Source: three-view drawing plus pictorial views. Frame: mm from the lowest corner of the part. A direction names the side the tool comes from. Coordinates: 2 decimals unless noted, no trailing zeros. Loops run counter-clockwise (first coordinate to the right, second up) from the corner with the lowest first, then second, coordinate; pieces in that order, holes last. Notation, with made-up numbers: (60, 74) - (91, 74) arc R13 ccw to (91, 94) - close; hole circle Ø4 at (42.25, 39). An arc over 180 degrees is marked (long way). Use CSV: the item, a comma, the result in double quotes. Start each with the question number.
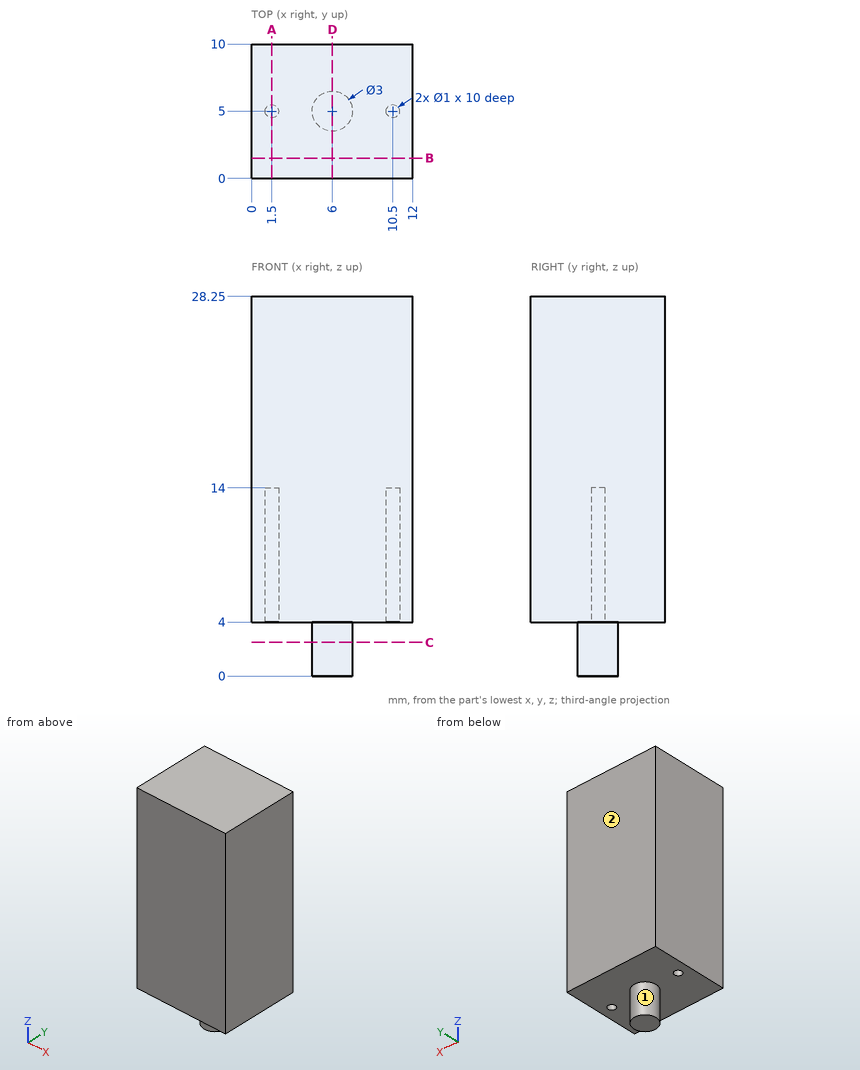
(1) Section A-A on x = 1.5. Output: boundary loops of the cut face in (y, z).
(2) Ray query, line 1 (Y direction, x = 1.5, z = 7.25); line 2 (Z direction, x = 8.5, y = 3.25); line 3 (Z direction, x = 10.25, y = 5). Return the intervals inside material, ascending. Write a range as [from, to].
(3) Pin query (flat end, axial travel): pin 1 Ø1 at (x, y) = (4.5, 3) entering from -Z; pin 2 Ø0.8 at (x, y) = (1.5, 5) entering from -Z. Return the tip coordinate at first contact, or that it passes through.
(4) Reachability of the marked faces 1 and 2 from +Z, -Z, +X, -X, +Y, -Y: full face, straight path, thin tool, end or side. Return the list, or none.
(5) Section B-B on y = 1.5. Output: boundary loops of the cut face in (x, z).
(6) Section D-D on x = 6. Output: boundary loops of the cut face in (y, z).
(7) Section C-C on z = 2.5. Output: boundary loops of the cut face in (x, y).
Solution:
1,outline,"(0, 4) - (4.5, 4) - (4.5, 14) - (5.5, 14) - (5.5, 4) - (10, 4) - (10, 28.25) - (0, 28.25) - close"
2,line 1,"y = [0, 4.5], [5.5, 10]"
2,line 2,"z = [4, 28.25]"
2,line 3,"z = [14, 28.25]"
3,pin 1,"stops at z = 4"
3,pin 2,"stops at z = 14"
4,face 1,"-Z"
4,face 2,"+Z, -Z, +X, -X, +Y"
5,outline,"(0, 4) - (12, 4) - (12, 28.25) - (0, 28.25) - close"
6,outline,"(0, 4) - (3.5, 4) - (3.5, 0) - (6.5, 0) - (6.5, 4) - (10, 4) - (10, 28.25) - (0, 28.25) - close"
7,outline,"circle Ø3 at (6, 5)"
